The listing builds one solid part. Answer for the finished solid, in the listing's coordinates (mm). A direction names the side the tool comes from. Coordinates: 2 decimals unless noted, no trailing zeros. Order: outer loops, then holes, each group sorted by start corner. A loop starts at its lowest first (then second) coordinate and runs counter-clockwise, first axis right, second up. Notation, with made-up numbers: (7.25, 11) - (11.25, 11) arc R23 cw to (11.25, 34) - close; hole circle Ø1 at (36, 52.25). An arc over 180 degrees is marked (long way). Use one line per item in the form item = value. Start each with the question number.
Item 1: Consider line 1 along Y through (x, z) = (0, 0.55); line 2 along X through (y, z) = (0.5, 1.95); line 3 along Y through (x, z) = (7, 0.45). Determine where each line is inside the solid, lowest interval first. Write a range as [from, to].
Item 2: Section A-A, the plane y = 0 is taken. Write down the section's boundary in (x, z).
Item 3: A tool of negligible diameter and unlimited length cuts with its end or side. For faces 5 (the cylindrical face through (-0.35, -8.56, 0.99)), 6 (the cylindrical face through (-0.54, -2.44, 3.48)), from which of +Z, -Z, +X, -X, +Y, -Y can it reach the whole face along a straight path? Write none if from no direction.
Item 4: Section B-B, the plane z = 0.75 is taken. Write down the section's boundary in (x, y), and give its area (3 significant figures).
Item 5: The mould has two halves that part along X. Classify faces 1 (the cylindrical face through (3.233, -1.341, 3.479)), 2 (the flat face through (0, 0, 2)), 3 (the cylindrical face through (5.4, 0.07, 0.99)), 4 (the flat face through (0, -4, 2)): released by +X, released by -X, zero draft, split by the parting line, or undercut.
Item 6: Each of these flat-tipped pins is pushed along its axis until it touches: pin 1 Ø3 at (x, z) = (3, 1) entering from -Y; pin 2 Ø2 at (x, z) = (6.5, 1.5) entering from +Y; pin 3 Ø1.5 at (x, y) = (-1, -1) entering from +Z. Where does it stop, or does it pass through?
Item 7: Section C-C, the plane y = 7 is taken. Write down the section's boundary in (x, z).
from build123d import *

# Parameters (mm, degrees)
SKETCH_1_R      = 10
SKETCH_1_R_2    = 1.6
EXTRUDE_1_DEPTH = 2
SKETCH_2_R      = 3.5
SKETCH_2_R_2    = 2.5
EXTRUDE_2_DEPTH = 3


with BuildPart() as part:
    # ｽｹｯﾁ1 → ﾎﾞｽ - 押し出し1 (new body)
    with BuildSketch(Plane.XY):
        Circle(SKETCH_1_R)
        with Locations((0, 7)):
            Circle(SKETCH_1_R_2, mode=Mode.SUBTRACT)
        with Locations((7, 0)):
            Circle(SKETCH_1_R_2, mode=Mode.SUBTRACT)
        with Locations((-7, 0)):
            Circle(SKETCH_1_R_2, mode=Mode.SUBTRACT)
        with Locations((0, -7)):
            Circle(SKETCH_1_R_2, mode=Mode.SUBTRACT)
    extrude(amount=EXTRUDE_1_DEPTH)

    # ｽｹｯﾁ2 → ﾎﾞｽ - 押し出し2 (add)
    with BuildSketch(Plane.XY.offset(2)):
        Circle(SKETCH_2_R)
        Circle(SKETCH_2_R_2, mode=Mode.SUBTRACT)
    extrude(amount=EXTRUDE_2_DEPTH)


solid = part.part
Response:
q1.line_1 = [-10, -8.6], [-5.4, 5.4], [8.6, 10]
q1.line_2 = [-9.99, -8.52], [-5.48, 5.48], [8.52, 9.99]
q1.line_3 = [-7.14, -1.6], [1.6, 7.14]
q2.outline = (-10, 0) - (-8.6, 0) - (-8.6, 2) - (-10, 2) - close; (-5.4, 0) - (5.4, 0) - (5.4, 2) - (3.5, 2) - (3.5, 5) - (2.5, 5) - (2.5, 2) - (-2.5, 2) - (-2.5, 5) - (-3.5, 5) - (-3.5, 2) - (-5.4, 2) - close; (8.6, 0) - (10, 0) - (10, 2) - (8.6, 2) - close
q3.face_5 = +Z, -Z
q3.face_6 = +Z
q4.outline = circle Ø20 at (0, 0); hole circle Ø3.2 at (-7, 0); hole circle Ø3.2 at (0, -7); hole circle Ø3.2 at (0, 7); hole circle Ø3.2 at (7, 0)
q4.area = 282 mm2
q5.face_1 = split by the parting line
q5.face_2 = undercut
q5.face_3 = undercut
q5.face_4 = zero draft
q6.pin_1 = -9.89
q6.pin_2 = 8.35
q6.pin_3 = 2
q7.outline = (-7.14, 0) - (-1.6, 0) - (-1.6, 2) - (-7.14, 2) - close; (1.6, 0) - (7.14, 0) - (7.14, 2) - (1.6, 2) - close
